For this review, take the finished solid that the model builds, in its own axes (mm). Face numbers are marked on the shaded views. A direction names the side the tool comes from. Coordinates: 2 decimals unless noted, no trailing zeros. Loops run counter-clockwise (first coordinate to the right, second up) from the corner with the lowest first, then second, coordinate; pieces in that order, holes last. Notation, with made-up numbers: (1, -17) - (13, -17) arc R13 ccw to (13, 7) - close; hole circle Ø5 at (66.5, 35.5). An arc over 180 degrees is marked (long way). Answer as a JSON object with one key per item and string values. Group by question number.
Item 1: We need section B-B (z = 3). Give the boundary of the cut face in (x, y), then the cut area to 3 significant figures.
Item 2: Tool access review of the marked faces 1 and 2: name each direction out of +Z, -Z, +X, -X, +Y, -Y from which nothing blocks a thin tool from reaching the whole face with its end or side.
Item 3: Mouldability with a two-part tool opening along X and no side actions: class the marked faces 3, 4 and 5 as released by +X, released by -X, zero draft, split by the parting line, or undercut.
Item 4: We need section C-C (x = 14.5). Give the boundary of the cut face in (y, z).
Item 5: We need section D-D (y = 1). Give the boundary of the cut face in (x, z), then the cut area to 3 significant figures.
Item 6: To check wall thickness, follow line 1 (Z direction, x = 13, y = -5.25); line 2 (X direction, y = 3.5, z = 3.5); line 3 (Y direction, x = 33, z = 0.5). State the ranges of each line that lie inside material, in increasing order.
Item 7: We need section A-A (y = -4.5). Give the boundary of the cut face in (x, z).
Item 8: Clearance check with flat-ended pins moving along their axes: pin 1 (1.2 mm diameter, centred on y = -2.5, z = 16, fed in from -X); pin 2 (6 mm diameter, centred on x = -4, z = 5.5, fed in from -Y); pin 3 (1.2 mm diameter, centred on x = -17.5, y = 3.5, fed in from +Z). State where each tip first meets the part, or that it passes through.
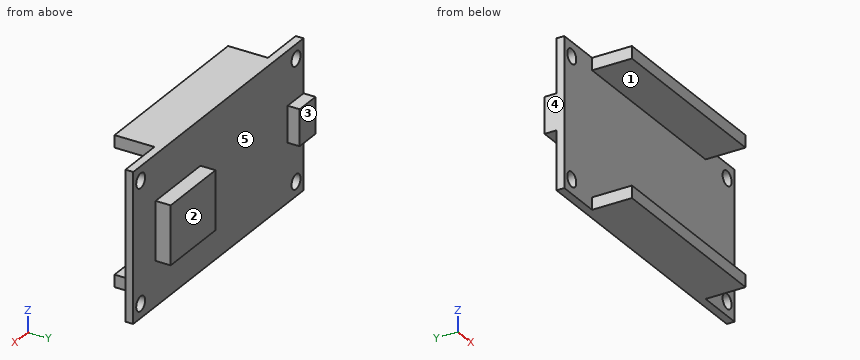
from build123d import *

# Parameters (mm, degrees)
SKETCH_1_W          = 57
SKETCH_1_H          = 30.4
EXTRUDE_1_DEPTH     = 1.6
SKETCH_2_W          = 15
SKETCH_2_H          = 12
EXTRUDE_2_DEPTH     = 3.1
SKETCH_3_W          = 5.3
SKETCH_3_H          = 7.4
EXTRUDE_3_DEPTH     = 2.46
SKETCH_4_R          = 1.5
CUT_EXTRUDE_1_DEPTH = 2.6
SKETCH_5_W          = 38
SKETCH_5_H          = 2.5
EXTRUDE_4_DEPTH     = 8.2


with BuildPart() as part:
    # 草图1 → 凸台-拉伸1 (new body)
    with BuildSketch(Plane(origin=(0, 0, 0), x_dir=(1, 0, 0), z_dir=(0, 1, 0))):
        with Locations((9.099869202, -2.04798995)):
            Rectangle(SKETCH_1_W, SKETCH_1_H)
    extrude(amount=EXTRUDE_1_DEPTH)

    # 草图2 → 凸台-拉伸2 (add)
    with BuildSketch(Plane(origin=(0, 1.6, 0), x_dir=(1, 0, 0), z_dir=(0, 1, 0))):
        with Locations((22.599869202, -1.94798995)):
            Rectangle(SKETCH_2_W, SKETCH_2_H)
    extrude(amount=EXTRUDE_2_DEPTH)

    # 草图3 → 凸台-拉伸3 (add)
    with BuildSketch(Plane(origin=(0, 1.6, 0), x_dir=(1, 0, 0), z_dir=(0, 1, 0))):
        with Locations((-16.750130798, -2.54798995)):
            Rectangle(SKETCH_3_W, SKETCH_3_H)
    extrude(amount=EXTRUDE_3_DEPTH)

    # 草图4 → 切除-拉伸1 (cut, through all)
    with BuildSketch(Plane(origin=(0, 1.6, 0), x_dir=(1, 0, 0), z_dir=(0, 1, 0))):
        with Locations((-16.900130798, 10.25201005)):
            Circle(SKETCH_4_R)
        with Locations((-16.900130798, -14.34798995)):
            Circle(SKETCH_4_R)
        with Locations((35.099869202, -14.34798995)):
            Circle(SKETCH_4_R)
        with Locations((35.099869202, 10.25201005)):
            Circle(SKETCH_4_R)
    extrude(amount=-CUT_EXTRUDE_1_DEPTH, mode=Mode.SUBTRACT)

    # 草图5 → 凸台-拉伸4 (add)
    with BuildSketch(Plane.XZ):
        with Locations((8.899869202, 15.99798995)):
            Rectangle(SKETCH_5_W, SKETCH_5_H)
        with Locations((8.899869202, -11.90201005)):
            Rectangle(SKETCH_5_W, SKETCH_5_H)
    extrude(amount=EXTRUDE_4_DEPTH)


solid = part.part
Check sheet entries:
{
 "1": {"outline": "(-19.4, 0) - (37.6, 0) - (37.6, 1.6) - (30.1, 1.6) - (30.1, 4.7) - (15.1, 4.7) - (15.1, 1.6) - (-14.1, 1.6) - (-14.1, 4.06) - (-19.4, 4.06) - close", "area": "151 mm2"},
 "2": {"face 1": "+X, -X, -Y", "face 2": "+Z, -Z, +X, -X, +Y"},
 "3": {"face 3": "zero draft", "face 4": "released by -X", "face 5": "undercut"},
 "4": {"outline": "(-8.2, -13.15) - (1.6, -13.15) - (1.6, 17.25) - (-8.2, 17.25) - (-8.2, 14.75) - (0, 14.75) - (0, -10.65) - (-8.2, -10.65) - close"},
 "5": {"outline": "(-19.4, -13.15) - (37.6, -13.15) - (37.6, 17.25) - (-19.4, 17.25) - close; hole circle Ø3 at (-16.9, -10.25); hole circle Ø3 at (-16.9, 14.35); hole circle Ø3 at (35.1, -10.25); hole circle Ø3 at (35.1, 14.35)", "area": "1,700 mm2"},
 "6": {"line 1": "z = -13.15 to -10.65, 14.75 to 17.25", "line 2": "x = -19.4 to -14.1, 15.1 to 30.1", "line 3": "y = 0 to 1.6"},
 "7": {"outline": "(-10.1, -13.15) - (27.9, -13.15) - (27.9, -10.65) - (-10.1, -10.65) - close; (-10.1, 14.75) - (27.9, 14.75) - (27.9, 17.25) - (-10.1, 17.25) - close"},
 "8": {"pin 1": "stops at x = -10.1", "pin 2": "stops at y = 0", "pin 3": "stops at z = 6.25"}
}
